Source: three-view drawing plus pictorial views. Frame: mm from the lowest corner of the part. Give positions to 0.01 mm unless a question says otherwise; leave off trailing zeros. Loops run counter-clockwise (first coordinate to the right, second up) from the corner with the lowest first, then second, coordinate; pieces in that order, holes last.
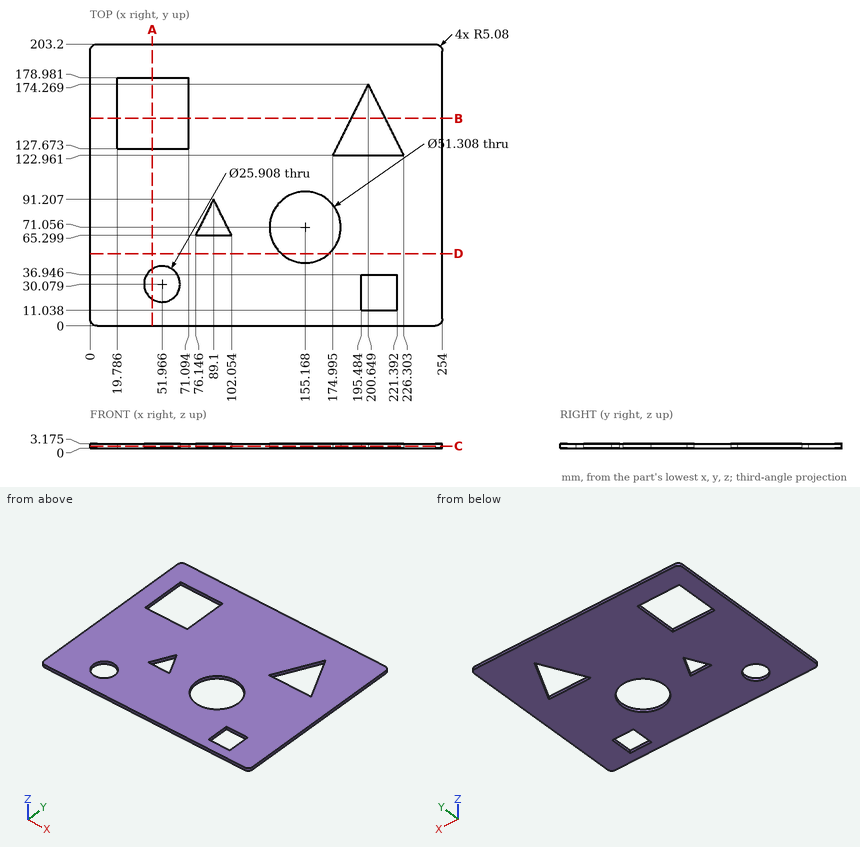
1) Cut plane B-B (y = 149.5). Return loops of the section in (x, z) (1 decimal).
Checks:
outline: (0, 0) - (19.8, 0) - (19.8, 3.2) - (0, 3.2) - close; (71.1, 0) - (188.3, 0) - (188.3, 3.2) - (71.1, 3.2) - close; (213, 0) - (254, 0) - (254, 3.2) - (213, 3.2) - close
2) Cut plane C-C (z = 1.4). Return loops of the section in (x, y) (1 decimal), and give its area (3 significant figures).
Checks:
outline: (0, 5.1) arc R5.1 ccw to (5.1, 0) - (248.9, 0) arc R5.1 ccw to (254, 5.1) - (254, 198.1) arc R5.1 ccw to (248.9, 203.2) - (5.1, 203.2) arc R5.1 ccw to (0, 198.1) - close; hole (19.8, 127.7) - (71.1, 127.7) - (71.1, 179) - (19.8, 179) - close; hole circle Ø25.9 at (52, 30.1); hole (76.1, 65.3) - (102.1, 65.3) - (89.1, 91.2) - close; hole circle Ø51.3 at (155.2, 71.1); hole (175, 123) - (226.3, 123) - (200.6, 174.3) - close; hole (195.5, 11) - (221.4, 11) - (221.4, 36.9) - (195.5, 36.9) - close
area: 44,000 mm2
3) Ray query, probe 1 along X at (y, z) = (174.5, 2.45) (1 decimal); probe 2 along Y at (x, z) = (175.5, 0.8) (1 decimal); probe 3 along Y at (x, z) = (62.5, 1.95) (1 decimal). Return the intervals inside material, ascending.
Checks:
probe 1: x = 0 to 19.8, 71.1 to 254
probe 2: y = 0 to 55.4, 86.7 to 123, 124 to 203.2
probe 3: y = 0 to 22.5, 37.6 to 127.7, 179 to 203.2
4) Contact query for a flat-ended pin moving along its axis: P1, Ø1, axis at x = 215, z = 1, coming from the -Y side. Output: stop coordinate, or through.
Checks:
P1: stops at y = 0
5) Cut plane D-D (y = 52). Return loops of the section in (x, z) (1 decimal).
Checks:
outline: (0, 0) - (138, 0) - (138, 3.2) - (0, 3.2) - close; (172.3, 0) - (254, 0) - (254, 3.2) - (172.3, 3.2) - close
6) Cut plane A-A (x = 45). Return loops of the section in (y, z) (1 decimal).
Checks:
outline: (0, 0) - (19.2, 0) - (19.2, 3.2) - (0, 3.2) - close; (41, 0) - (127.7, 0) - (127.7, 3.2) - (41, 3.2) - close; (179, 0) - (203.2, 0) - (203.2, 3.2) - (179, 3.2) - close
